Answer from the drawing. Dimensions are ordinates in mm from the lowest x, y and z of the part. Give positions to 0.01 mm unless a question says otherwise; leave off trailing zeros. Loops run counter-clockwise (first coordinate to the right, second up) from the corner with the lowest first, then second, coordinate; pieces in that order, holes last. Notation, with made-up numbers: (67.5, 73) - (121.5, 73) arc R24 ccw to (121.5, 90) - close; hole circle Ø2 at (64, -15). An arc over 180 degrees is marked (long way). Write each question's results on one line, items separated by ' | '. Start each with the question number.
Q1. The part is cut by section A-A, the plane y = 17. Write down the section's boundary in (x, z), plus the area to 3 significant figures.
Q2. Given pin 1 (4 mm diameter, centred on y = 37.5, z = 12, fed in from +X); pin 2 (8 mm diameter, centred on y = 45, z = 28.5, fed in from -X); pin 3 (3 mm diameter, centred on x = 14, y = 26, fed in from +Z), each flat-ended and moving along its own axis, determine where each tip first touches the part or whether it passes through.
Q3. Find the intervals of material crossed by line 1 (Z direction, x = 2, y = 24.5); line 2 (X direction, y = 50, z = 31.5); line 3 (X direction, y = 7, z = 4.5), in increasing order. Write a range as from..to.
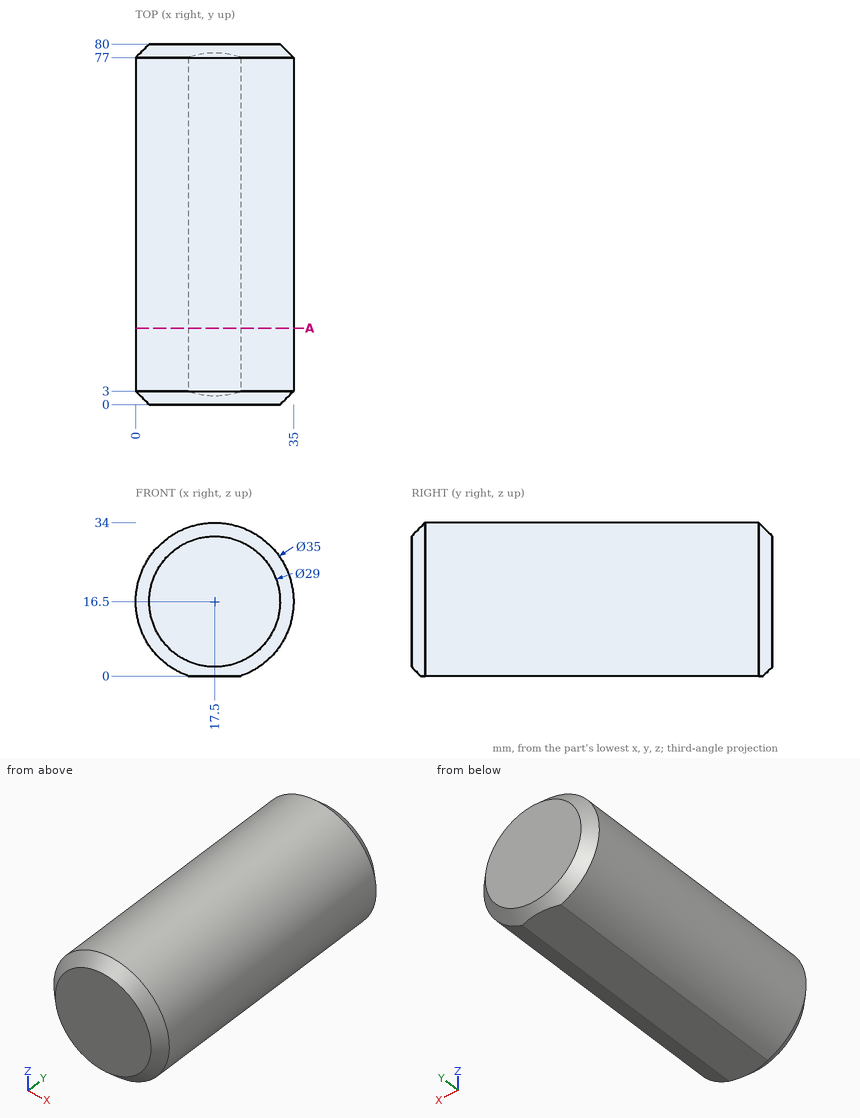
Check sheet entries:
1) outline: (11.67, 0) - (23.33, 0) arc R17.5 ccw (long way) to start | area: 954 mm^2
2) pin 1: stops at x = 34.82 | pin 2: stops at x = 1.94 | pin 3: stops at z = 33.89
3) line 1: z = 8.38..24.62 | line 2: x = 8.49..26.51 | line 3: x = 4.76..30.24
